```python
from build123d import *

# Parameters (mm, degrees)
CROQUIS1_W                      = 93
CROQUIS1_H                      = 87
SALIENTE_EXTRUIR1_DEPTH         = 1.5
DI_METRO_DE_TALADRO_3_1_3_1_1_D = 3.1
CROQUIS9_R                      = 3
SALIENTE_EXTRUIR4_DEPTH         = 24


with BuildPart() as part:
    # Croquis1 → Saliente-Extruir1 (new body)
    with BuildSketch(Plane(origin=(0, 0, 0), x_dir=(-1, 0, 0), z_dir=(0, 0, -1))):
        Rectangle(CROQUIS1_W, CROQUIS1_H)
    extrude(amount=-SALIENTE_EXTRUIR1_DEPTH)

    # Diámetro de taladro Ø3.1 (3.1)1 (through all)
    with Locations(Plane(origin=(0, 0, 0), x_dir=(-1, 0, 0), z_dir=(0, 0, -1))):
        with Locations((43.95, -23.95), (-43.95, -23.95), (43.95, 40.95), (-43.95, 40.95)):
            Hole(DI_METRO_DE_TALADRO_3_1_3_1_1_D / 2)

    # Croquis9 → Saliente-Extruir4 (add)
    with BuildSketch(Plane.XY.offset(1.5)):
        with Locations(Location((31.1, -33.5, 0), (0, 0, 180))):
            Circle(CROQUIS9_R)
    extrude(amount=SALIENTE_EXTRUIR4_DEPTH)


solid = part.part
```
Geometry: final body of the model. Coordinates: model frame, mm. Coordinates: 2 decimals unless noted, no trailing zeros. Write each loop counter-clockwise with the first axis right and the second up, starting at its lowest first coordinate (ties: lowest second). Pieces come first, ordered by that corner, then holes. Notation, with made-up numbers: M -36.5,18 L -24.5,18 A27 cw -24.5,54 Z; hole C 50.5,-27.75 d4. An arc over 180 degrees is marked long. Use CSV: the item, a comma, the result in double quotes. Start each with the question number.
1. Cut plane B-B on x = 43.95. Return the cut outline in (y, z).
2. Ray query, probe 1 along Y at (x, z) = (43.95, 0.35); probe 2 along Z at (x, y) = (-28.5, -9); probe 3 along X at (y, z) = (-33, 18). Return the intervals inside material, ascending.
3. Mould query, pull axis Y, two halves, no side actions, for faces 1 (the face through (31.491, -36.474, 13.332)), 2 (the face through (1, 1, 1.5)), 3 (the face through (-45.09, 42, 0.76)). Classes: pulls with the +Y half, pulls with the -Y half, needs draft (parallel to the pull), parting line crosses it, or undercut.
4. First-contact query: P1, Ø6, axis at x = 5, y = 18, coming from the +Z side; P2, Ø12, axis at y = -17.5, z = 12.5, coming from the +X side. Flat tips, straight axial feed; report the tip coordinate or a pass-through.
5. Cut plane A-A on y = -23.95. Return the cut outline in (x, z), plus the area to 3 significant figures.
6. Cut plane D-D on z = 14. Return the cut outline in (x, y).
7. Cut plane C-C on x = 31.1. Return the cut outline in (y, z), plus the area to 4 significant figures.
Entries:
1,outline,"M -43.5,0 L -25.5,0 L -25.5,1.5 L -43.5,1.5 Z; M -22.4,0 L 39.4,0 L 39.4,1.5 L -22.4,1.5 Z; M 42.5,0 L 43.5,0 L 43.5,1.5 L 42.5,1.5 Z"
2,probe 1,"-43.5 to -25.5, -22.4 to 39.4, 42.5 to 43.5"
2,probe 2,"0 to 1.5"
2,probe 3,"28.14 to 34.06"
3,face 1,"parting line crosses it"
3,face 2,"needs draft"
3,face 3,"undercut"
4,P1,"z = 1.5"
4,P2,"through"
5,outline,"M -46.5,0 L -45.5,0 L -45.5,1.5 L -46.5,1.5 Z; M -42.4,0 L 42.4,0 L 42.4,1.5 L -42.4,1.5 Z; M 45.5,0 L 46.5,0 L 46.5,1.5 L 45.5,1.5 Z"
5,area,"130 mm²"
6,outline,"C 31.1,-33.5 d6"
7,outline,"M -43.5,0 L 43.5,0 L 43.5,1.5 L -30.5,1.5 L -30.5,25.5 L -36.5,25.5 L -36.5,1.5 L -43.5,1.5 Z"
7,area,"274.5 mm²"
